Check sheet for the modelled part. Datum: model origin and axes. Units: mm. Give positions to 0.01 mm unless a question says otherwise; leave off trailing zeros. Order: outer loops, then holes, each group sorted by start corner. A loop starts at its lowest first (then second) coordinate and runs counter-clockwise, first axis right, second up.
```python
from build123d import *

# Parameters (mm, degrees)
SKETCH1_W              = 76.2
SKETCH1_H              = 40.64
BASE_FLANGE1_DEPTH     = 2.286
CUT_EXTRUDE1_REACH     = 249.845
SKETCH6_R              = 2.5527
SKETCH6_R_2            = 3.175
FILLET1_R              = 3.175
SKETCH7_W              = 53.484881044
SKETCH7_H              = 41.537228889
REMOVE_3RD_STAGE_DEPTH = 2.54
FILLET2_R              = 3.175
SKETCH8_W              = 26.577580406
SKETCH8_H              = 64.780145769
REMOVE_2ND_STAGE_DEPTH = 248.845041068
FILLET3_R              = 3.175


# Sheet-metal steps are written as plain solids
with BuildPart() as part:
    # Sketch1 → Base-Flange1 (new body)
    with BuildSketch(Plane.XY):
        with Locations((-119.218460544, -171.181541922)):
            Rectangle(SKETCH1_W, SKETCH1_H)
    extrude(amount=BASE_FLANGE1_DEPTH)

    # Sketch6 → Cut-Extrude1 (cut, up to next)
    with BuildSketch(Plane(origin=(0, 0, 0), x_dir=(-1, 0, 0), z_dir=(0, 0, -1)), mode=Mode.PRIVATE) as cut_extrude1_sk1:
        with Locations((150.6232, -158.481541922)):
            Circle(SKETCH6_R)
    cut_extrude1_tool1 = extrude(cut_extrude1_sk1.sketch, amount=-CUT_EXTRUDE1_REACH, mode=Mode.PRIVATE) & part.part
    # Sketch6 → Cut-Extrude1 (cut, up to next)
    with BuildSketch(Plane(origin=(0, 0, 0), x_dir=(-1, 0, 0), z_dir=(0, 0, -1)), mode=Mode.PRIVATE) as cut_extrude1_sk2:
        with Locations((150.6232, -183.881541922)):
            Circle(SKETCH6_R)
    cut_extrude1_tool2 = extrude(cut_extrude1_sk2.sketch, amount=-CUT_EXTRUDE1_REACH, mode=Mode.PRIVATE) & part.part
    # Sketch6 → Cut-Extrude1 (cut, up to next)
    with BuildSketch(Plane(origin=(0, 0, 0), x_dir=(-1, 0, 0), z_dir=(0, 0, -1)), mode=Mode.PRIVATE) as cut_extrude1_sk3:
        with Locations((118.4918, -158.481541922)):
            Circle(SKETCH6_R)
    cut_extrude1_tool3 = extrude(cut_extrude1_sk3.sketch, amount=-CUT_EXTRUDE1_REACH, mode=Mode.PRIVATE) & part.part
    # Sketch6 → Cut-Extrude1 (cut, up to next)
    with BuildSketch(Plane(origin=(0, 0, 0), x_dir=(-1, 0, 0), z_dir=(0, 0, -1)), mode=Mode.PRIVATE) as cut_extrude1_sk4:
        with Locations((119.9918, -171.181541922)):
            Circle(SKETCH6_R_2)
    cut_extrude1_tool4 = extrude(cut_extrude1_sk4.sketch, amount=-CUT_EXTRUDE1_REACH, mode=Mode.PRIVATE) & part.part
    # Sketch6 → Cut-Extrude1 (cut, up to next)
    with BuildSketch(Plane(origin=(0, 0, 0), x_dir=(-1, 0, 0), z_dir=(0, 0, -1)), mode=Mode.PRIVATE) as cut_extrude1_sk5:
        with Locations((118.4918, -183.881541922)):
            Circle(SKETCH6_R)
    cut_extrude1_tool5 = extrude(cut_extrude1_sk5.sketch, amount=-CUT_EXTRUDE1_REACH, mode=Mode.PRIVATE) & part.part
    # Sketch6 → Cut-Extrude1 (cut, up to next)
    with BuildSketch(Plane(origin=(0, 0, 0), x_dir=(-1, 0, 0), z_dir=(0, 0, -1)), mode=Mode.PRIVATE) as cut_extrude1_sk6:
        with Locations((131.1918, -158.481541922)):
            Circle(SKETCH6_R)
    cut_extrude1_tool6 = extrude(cut_extrude1_sk6.sketch, amount=-CUT_EXTRUDE1_REACH, mode=Mode.PRIVATE) & part.part
    # Sketch6 → Cut-Extrude1 (cut, up to next)
    with BuildSketch(Plane(origin=(0, 0, 0), x_dir=(-1, 0, 0), z_dir=(0, 0, -1)), mode=Mode.PRIVATE) as cut_extrude1_sk7:
        with Locations((132.6918, -171.181541922)):
            Circle(SKETCH6_R_2)
    cut_extrude1_tool7 = extrude(cut_extrude1_sk7.sketch, amount=-CUT_EXTRUDE1_REACH, mode=Mode.PRIVATE) & part.part
    # Sketch6 → Cut-Extrude1 (cut, up to next)
    with BuildSketch(Plane(origin=(0, 0, 0), x_dir=(-1, 0, 0), z_dir=(0, 0, -1)), mode=Mode.PRIVATE) as cut_extrude1_sk8:
        with Locations((131.1918, -183.881541922)):
            Circle(SKETCH6_R)
    cut_extrude1_tool8 = extrude(cut_extrude1_sk8.sketch, amount=-CUT_EXTRUDE1_REACH, mode=Mode.PRIVATE) & part.part
    # Sketch6 → Cut-Extrude1 (cut, up to next)
    with BuildSketch(Plane(origin=(0, 0, 0), x_dir=(-1, 0, 0), z_dir=(0, 0, -1)), mode=Mode.PRIVATE) as cut_extrude1_sk9:
        with Locations((105.7918, -158.481541922)):
            Circle(SKETCH6_R)
    cut_extrude1_tool9 = extrude(cut_extrude1_sk9.sketch, amount=-CUT_EXTRUDE1_REACH, mode=Mode.PRIVATE) & part.part
    # Sketch6 → Cut-Extrude1 (cut, up to next)
    with BuildSketch(Plane(origin=(0, 0, 0), x_dir=(-1, 0, 0), z_dir=(0, 0, -1)), mode=Mode.PRIVATE) as cut_extrude1_sk10:
        with Locations((107.2918, -171.181541922)):
            Circle(SKETCH6_R_2)
    cut_extrude1_tool10 = extrude(cut_extrude1_sk10.sketch, amount=-CUT_EXTRUDE1_REACH, mode=Mode.PRIVATE) & part.part
    # Sketch6 → Cut-Extrude1 (cut, up to next)
    with BuildSketch(Plane(origin=(0, 0, 0), x_dir=(-1, 0, 0), z_dir=(0, 0, -1)), mode=Mode.PRIVATE) as cut_extrude1_sk11:
        with Locations((105.7918, -183.881541922)):
            Circle(SKETCH6_R)
    cut_extrude1_tool11 = extrude(cut_extrude1_sk11.sketch, amount=-CUT_EXTRUDE1_REACH, mode=Mode.PRIVATE) & part.part
    # Sketch6 → Cut-Extrude1 (cut, up to next)
    with BuildSketch(Plane(origin=(0, 0, 0), x_dir=(-1, 0, 0), z_dir=(0, 0, -1)), mode=Mode.PRIVATE) as cut_extrude1_sk12:
        with Locations((93.0918, -158.481541922)):
            Circle(SKETCH6_R)
    cut_extrude1_tool12 = extrude(cut_extrude1_sk12.sketch, amount=-CUT_EXTRUDE1_REACH, mode=Mode.PRIVATE) & part.part
    # Sketch6 → Cut-Extrude1 (cut, up to next)
    with BuildSketch(Plane(origin=(0, 0, 0), x_dir=(-1, 0, 0), z_dir=(0, 0, -1)), mode=Mode.PRIVATE) as cut_extrude1_sk13:
        with Locations((94.5918, -171.181541922)):
            Circle(SKETCH6_R_2)
    cut_extrude1_tool13 = extrude(cut_extrude1_sk13.sketch, amount=-CUT_EXTRUDE1_REACH, mode=Mode.PRIVATE) & part.part
    # Sketch6 → Cut-Extrude1 (cut, up to next)
    with BuildSketch(Plane(origin=(0, 0, 0), x_dir=(-1, 0, 0), z_dir=(0, 0, -1)), mode=Mode.PRIVATE) as cut_extrude1_sk14:
        with Locations((93.0918, -183.881541922)):
            Circle(SKETCH6_R)
    cut_extrude1_tool14 = extrude(cut_extrude1_sk14.sketch, amount=-CUT_EXTRUDE1_REACH, mode=Mode.PRIVATE) & part.part
    add(cut_extrude1_tool1.solids().sort_by_distance((-150.6232, -158.481542, 0))[0], mode=Mode.SUBTRACT)
    add(cut_extrude1_tool2.solids().sort_by_distance((-150.6232, -183.881542, 0))[0], mode=Mode.SUBTRACT)
    add(cut_extrude1_tool3.solids().sort_by_distance((-118.4918, -158.481542, 0))[0], mode=Mode.SUBTRACT)
    add(cut_extrude1_tool4.solids().sort_by_distance((-119.9918, -171.181542, 0))[0], mode=Mode.SUBTRACT)
    add(cut_extrude1_tool5.solids().sort_by_distance((-118.4918, -183.881542, 0))[0], mode=Mode.SUBTRACT)
    add(cut_extrude1_tool6.solids().sort_by_distance((-131.1918, -158.481542, 0))[0], mode=Mode.SUBTRACT)
    add(cut_extrude1_tool7.solids().sort_by_distance((-132.6918, -171.181542, 0))[0], mode=Mode.SUBTRACT)
    add(cut_extrude1_tool8.solids().sort_by_distance((-131.1918, -183.881542, 0))[0], mode=Mode.SUBTRACT)
    add(cut_extrude1_tool9.solids().sort_by_distance((-105.7918, -158.481542, 0))[0], mode=Mode.SUBTRACT)
    add(cut_extrude1_tool10.solids().sort_by_distance((-107.2918, -171.181542, 0))[0], mode=Mode.SUBTRACT)
    add(cut_extrude1_tool11.solids().sort_by_distance((-105.7918, -183.881542, 0))[0], mode=Mode.SUBTRACT)
    add(cut_extrude1_tool12.solids().sort_by_distance((-93.0918, -158.481542, 0))[0], mode=Mode.SUBTRACT)
    add(cut_extrude1_tool13.solids().sort_by_distance((-94.5918, -171.181542, 0))[0], mode=Mode.SUBTRACT)
    add(cut_extrude1_tool14.solids().sort_by_distance((-93.0918, -183.881542, 0))[0], mode=Mode.SUBTRACT)

    # Fillet1
    fillet1_edges = [part.edges().sort_by_distance(p)[0] for p in [
        (-157.318460544, -150.861541922, 1.143),
        (-81.118460544, -150.861541922, 1.143),
        (-81.118460544, -191.501541922, 1.143),
        (-157.318460544, -191.501541922, 1.143),
    ]]
    fillet(fillet1_edges, radius=FILLET1_R)

    # Sketch7 → Remove 3rd Stage (cut)
    with BuildSketch(Plane.XY.offset(2.286)):
        with Locations((-75.050259478, -170.732927477)):
            Rectangle(SKETCH7_W, SKETCH7_H)
    extrude(amount=-REMOVE_3RD_STAGE_DEPTH, mode=Mode.SUBTRACT)

    # Fillet2
    fillet2_edges = [part.edges().sort_by_distance(p)[0] for p in [
        (-101.7927, -150.861541922, 1.143),
        (-101.7927, -191.501541922, 1.143),
    ]]
    fillet(fillet2_edges, radius=FILLET2_R)

    # Sketch8 → Remove 2nd Stage (cut, through all)
    with BuildSketch(Plane.XY.offset(2.286)):
        with Locations((-101.203909797, -170.174492323)):
            Rectangle(SKETCH8_W, SKETCH8_H)
    extrude(amount=-REMOVE_2ND_STAGE_DEPTH, mode=Mode.SUBTRACT)

    # Fillet3
    fillet3_edges = [part.edges().sort_by_distance(p)[0] for p in [
        (-114.4927, -191.501541922, 1.143),
        (-114.4927, -150.861541922, 1.143),
    ]]
    fillet(fillet3_edges, radius=FILLET3_R)


solid = part.part
```
(1) Material ranges on L1, parallel to Y at x = -130, z = 1.45; L2, parallel to Y at x = -132, z = 0.9; L3, parallel to Y at x = -149.5, z = 0.95, recorded low to high.
Response values:
L1: y = -191.5 to -186.14, -181.62 to -172.87, -169.5 to -160.74, -156.22 to -150.86
L2: y = -191.5 to -186.3, -181.46 to -174.28, -168.08 to -160.9, -156.06 to -150.86
L3: y = -191.5 to -186.17, -181.59 to -160.77, -156.19 to -150.86
(2) Cross-section at B-B on y = -160. Enter the section's corners in (x, z), then the cut area to 3 significant figures.
Response values:
outline: (-157.32, 0) - (-152.68, 0) - (-152.68, 2.29) - (-157.32, 2.29) - close; (-148.57, 0) - (-133.24, 0) - (-133.24, 2.29) - (-148.57, 2.29) - close; (-129.14, 0) - (-120.54, 0) - (-120.54, 2.29) - (-129.14, 2.29) - close; (-116.44, 0) - (-114.49, 0) - (-114.49, 2.29) - (-116.44, 2.29) - close
area: 69.8 mm2
(3) Cross-section at A-A on z = 0.5. Count the separate pieces of the cut face and the enclosed holes in it, then the cut area to 3 significant figures.
Response values:
separate pieces: 1
enclosed holes: 8
area: 1,550 mm2
(4) Release check for a two-part mould opening along X. For faces 1 (the face through (-114.493, -171, 1)), 2 (the face through (-136.2, -170.9, 0)), 3 (the face through (-130.638, -160.974, 1.127)), 4 (the face through (-157.318, -171, 1)) record: released by +X, released by -X, zero draft, split by the parting line, or undercut.
Response values:
face 1: released by +X
face 2: zero draft
face 3: undercut
face 4: released by -X
